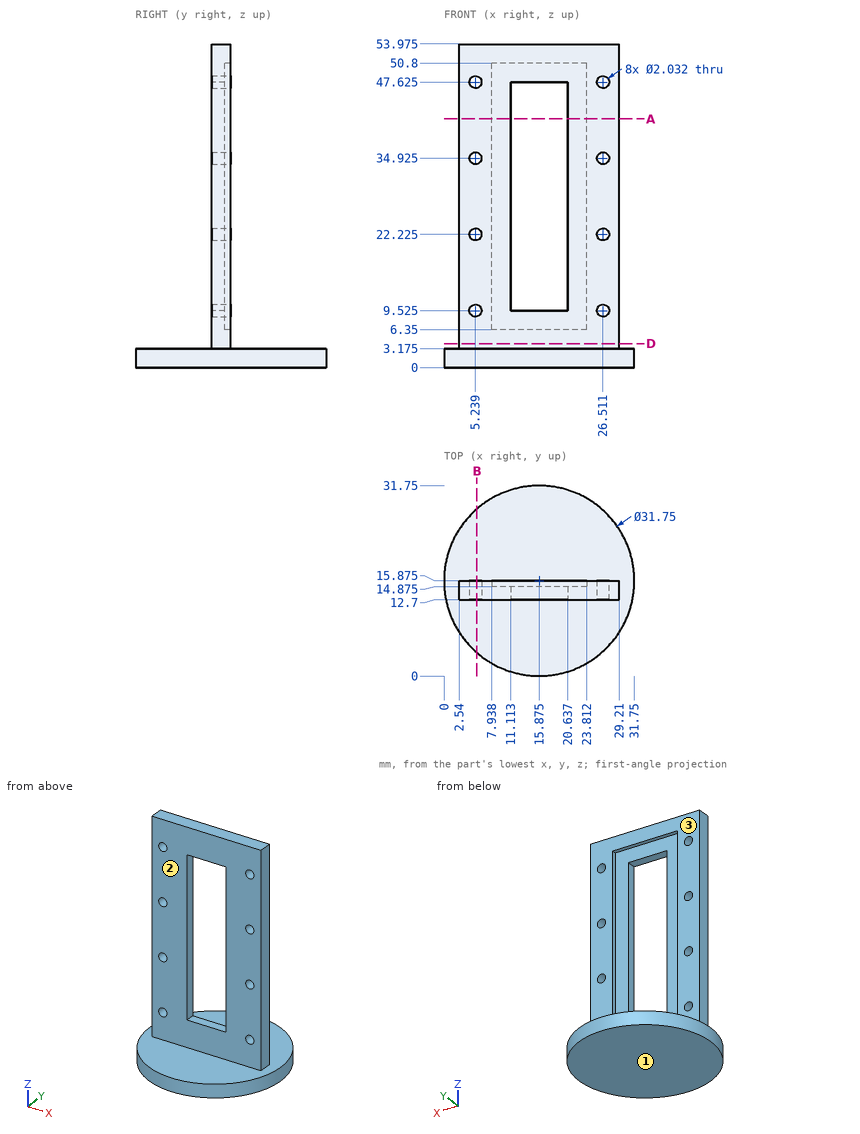
Part print with two shaded views. Sizes in mm from the minimum x, y, z corner. A direction names the side the tool comes from. Coordinates: 2 decimals unless noted, no trailing zeros. Order: outer loops, then holes, each group sorted by start corner. A loop starts at its lowest first (then second) coordinate and runs counter-clockwise, first axis right, second up. Notation, with made-up numbers: (5.5, 80) - (51.5, 80) arc R26 cw to (51.5, 107) - close; hole circle Ø3 at (-29, 83.25). An arc over 180 degrees is marked (long way). Write item = value, one per line. Start each with the question number.
1) 3-axis set-ups, long thin cutter, end or side, ignore diameter. For the marked faces 1, 2 and 3: which of +Z, -Z, +X, -X, +Y, -Y reach the whole face in a straight line?
2) Saw through at A-A on z = 41.5. Write the cut outline in (x, y) (1 decimal).
3) Saw through at D-D on z = 4. Write the cut outline in (x, y) (1 decimal).
4) Flat gauge pins, fed straight in: pin 1 Ø5 at (x, y) = (9, 4) entering from +Z (1 decimal); pin 2 Ø2.5 at (x, z) = (26.51, 34.92) entering from -Y; pin 3 Ø0.8 at (y, z) = (15.5, 35.5) entering from -X; pin 4 Ø1.2 at (x, z) = (26.51, 47.62) entering from +Y. Where does each tip first touch, or does it go through?
5) Saw through at B-B on x = 5.5. Write the cut outline in (y, z) (1 decimal).
6) Wall check: line 1 along X through (y, z) = (15, 16); line 2 along Y through (x, z) = (23, 16.5) (1 decimal); line 3 along Y through (x, z) = (28.5, 49) (1 decimal). Give the ranges that are in metal, low to high. Write a range as from..to.
From the geometry:
q1.face_1 = -Z, +X, -X, +Y, -Y
q1.face_2 = +Z, +X, -X, -Y
q1.face_3 = +Z, +X, -X, +Y
q2.outline = (2.5, 12.7) - (11.1, 12.7) - (11.1, 14.9) - (7.9, 14.9) - (7.9, 15.9) - (2.5, 15.9) - close; (20.6, 12.7) - (29.2, 12.7) - (29.2, 15.9) - (23.8, 15.9) - (23.8, 14.9) - (20.6, 14.9) - close
q3.outline = (2.5, 12.7) - (29.2, 12.7) - (29.2, 15.9) - (2.5, 15.9) - close
q4.pin_1 = 3.2
q4.pin_2 = 12.7
q4.pin_3 = 2.54
q4.pin_4 = through
q5.outline = (3.9, 0) - (27.9, 0) - (27.9, 3.2) - (15.9, 3.2) - (15.9, 8.5) - (12.7, 8.5) - (12.7, 3.2) - (3.9, 3.2) - close; (12.7, 10.5) - (15.9, 10.5) - (15.9, 21.2) - (12.7, 21.2) - close; (12.7, 23.2) - (15.9, 23.2) - (15.9, 33.9) - (12.7, 33.9) - close; (12.7, 35.9) - (15.9, 35.9) - (15.9, 46.6) - (12.7, 46.6) - close; (12.7, 48.6) - (15.9, 48.6) - (15.9, 54) - (12.7, 54) - close
q6.line_1 = 2.54..7.94, 23.81..29.21
q6.line_2 = 12.7..14.9
q6.line_3 = 12.7..15.9
